Autodesk Inventor part; units mm, degrees
ref_plane "YZ Plane" through (0, 0, 0) normal (1, 0, 0) x (0, 1, 0)
ref_plane "XZ Plane" through (0, 0, 0) normal (0, 1, 0) x (-1, 0, 0)
ref_plane "XY Plane" through (0, 0, 0) normal (0, 0, 1) x (1, 0, 0)
sketch "Sketch1" plane through (0, 0, 0) normal (0, 1, 0) x (-1, 0, 0)
  line L0 (0, 0) -> (0, -45)
  line L1 (0, -45) -> (35, -45)
  line L2 (35, -45) -> (35, -49)
  line L3 (35, -49) -> (-4, -49)
  line L4 (-4, -49) -> (-4, 0)
  line L5 (-4, 0) -> (0, 0)
  dimension "d0" = 45
  dimension "d1" = 35
  dimension "d2" = 4
  dimension "d3" = 39
extrude "Extrusion1" add sketch "Sketch1" along normal blind 21
sketch "Sketch2" plane through (4, 0, 0) normal (1, 0, 0) x (0, 0, -1)
  line L0 (0, 21) -> (49, 21)
  line L1 (0, 21) -> (12.5, 21)
  line L2 (12.5, 21) -> (12.5, 16)
  line L3 (12.5, 16) -> (0, 16)
  line L4 (0, 16) -> (0, 21)
  line L5 (12.5, 16) -> (23.5, 16)
  line L6 (23.5, 16) -> (23.5, 5)
  line L7 (23.5, 5) -> (12.5, 5)
  line L8 (12.5, 5) -> (12.5, 16)
  circle A0 centre (12.5, 16) radius 1.5
  circle A1 centre (23.5, 16) radius 1.5
  circle A2 centre (12.5, 5) radius 1.5
  circle A3 centre (23.5, 5) radius 1.5
  point P0 (0, 0)
  dimension "d6" = 12.5
  dimension "d7" = 5
  dimension "d8" = 11
  dimension "d9" = 11
  dimension "d10" = 3
  dimension "d11" = 3
  dimension "d12" = 3
  dimension "d13" = 3
extrude "Extrusion2" cut sketch "Sketch2" against normal blind 21 contours A0 L5 L2 | L2 L3 A0 | L3 L8 A0 | L5 A0 L8 | A1 L6 L5 | L5 L6 A1 | A2 L7 L8 | L8 L7 A2 | A3 L7 L6 | L6 L7 A3
sketch "Sketch3" plane through (-35, 0, -45) normal (0, 0, 1) x (1, 0, 0)
  line L0 (0, 0) -> (0, 21)
  line L1 (0, 10.5) -> (10.5, 10.5)
  circle A0 centre (10.5, 10.5) radius 10.5
  line L2 (0, 21) -> (10.5, 21)
  line L3 (10.5, 21) -> (10.5, 0)
  line L4 (10.5, 0) -> (0, 0)
  line L5 (0, 0) -> (0, 21)
  circle A1 centre (10.5, 10.5) radius 8
  circle A2 centre (10.5, 10.5) radius 6.5
  line L6 (10.5, 18.5) -> (10.5, 17)
  line L7 (10.5, 4) -> (10.5, 2.5)
  line L8 (2.5, 10.5) -> (4, 10.5)
  line L9 (10.5, 10.5) -> (18.5, 10.5)
  line L10 (18.5, 10.5) -> (17, 10.5)
  circle A3 centre (10.5, 17.75) radius 1.1
  circle A4 centre (3.25, 10.5) radius 1.1
  circle A5 centre (17.75, 10.5) radius 1.1
  circle A6 centre (10.5, 3.25) radius 1.1
  circle A7 centre (10.5, 10.5) radius 3
  point P0 (35, 0)
  point P1 (10.5, 21)
  dimension "d16" = 10.5
  dimension "d17" = 16
  dimension "d18" = 13
  dimension "d19" = 2.2
  dimension "d20" = 2.2
  dimension "d21" = 2.2
  dimension "d22" = 2.2
  dimension "d23" = 6
extrude "Extrusion3" cut sketch "Sketch3" against normal blind 21 contours L0 A0 L4 | L0 L2 A0 | A4 A1 L1 | L1 A1 A4 | A6 A1 L3 | L3 A1 A6 | A1 A4 A2 L1 | L1 A2 A4 A1 | A3 A1 L3 | L3 A1 A3 | A1 A6 A2 L3 | L3 A2 A6 A1 | A2 A4 L1 | L1 A4 A2 | A1 L3 A2 A3 | A1 A3 A2 L3 | A2 A6 L3 | L3 A6 A2 | A5 A2 L9 A1 | A1 A5 | A2 L3 A3 | A2 A3 L3 | A1 L9 A2 A5 | A5 L9 A2 | A7 L3 L1 | L1 L3 A7 | A2 L9 A5 | L3 L9 A7 | L3 A7 L9
fillet "Fillet1" radius 4 1 edges at (0, 10.5, -45)
properties part number "L2"
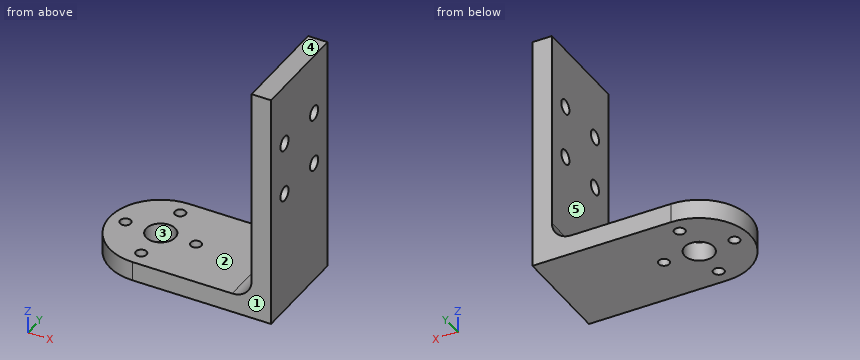
The listing builds one solid part. Answer for the finished solid, in the listing's coordinates (mm). Face numbers are marked on the shaded views. A direction names the side the tool comes from. Coordinates: 2 decimals unless noted, no trailing zeros. Loops run counter-clockwise (first coordinate to the right, second up) from the corner with the lowest first, then second, coordinate; pieces in that order, holes last. Notation, with made-up numbers: M -14,88 L 19,88 A19 ccw 19,106 Z; hole C -16.5,73.25 d8. An arc over 180 degrees is marked long. Answer as CSV lines item,"result". Start each with the question number.
(1) Find the intervals of material crossed by L1, parallel to X at y = 10.5, z = -47.15; L2, parallel to Y at x = -24.5, z = -46.5; L3, parallel to Y at x = 2.55, z = -23.5, in increasing order. Write a range as [from, to].
(2) The part is cut by section B-B (z = -12.5). Give the vertices of the cut face in (x, y).
(3) The part is cut by section C-C (x = -17.25). Give the vertices of the cut face in (y, z), and give its area (3 significant figures).
(4) Given pin 1 (2 mm diameter, centred on x = -31.75, y = 10.5, fed in from -Z); pin 2 (3 mm diameter, centred on x = -24.5, y = 3.25, fed in from +Z); pin 3 (12 mm diameter, centred on x = -7.5, y = 2, fed in from +Z); pin 4 (3.5 mm diameter, centred on y = 16, z = -12.5, fed in from -X), each flat-ended and moving along its own axis, determine where each tip first touches the part or whether it passes through.
(5) The part is cut by section A-A (y = 10.5). Give the vertices of the cut face in (x, z), and give its area (3 significant figures).
(6) For the marked faces 1 and 2, determine the directions among +Z, -Z, +X, -X, +Y, -Y from which every point of the face is accessible in a straight line to the end or side of a thin tool.
(7) The mould has two halves that part along X. Classify the marked faces 3, 4 and 5: pulls with the +X half, pulls with the -X half, needs draft (parallel to the pull), parting line crosses it, or undercut.
(8) The part is cut by section D-D (y = 19.5). Give the vertices of the cut face in (x, z), and give its area (3 significant figures).
Determined:
1,L1,"[-35, -32.85], [-30.65, -27.5], [-21.5, -18.35], [-16.15, 4]"
1,L2,"[0, 2.15], [4.35, 7.5], [13.5, 16.65], [18.85, 21]"
1,L3,"[0, 3.5], [6.5, 14.5], [17.5, 21]"
2,outline,"M 0,0 L 4,0 L 4,3.5 L 0,3.5 Z; M 0,6.5 L 4,6.5 L 4,14.5 L 0,14.5 Z; M 0,17.5 L 4,17.5 L 4,21 L 0,21 Z"
3,outline,"M 0,-49 L 9.4,-49 L 9.4,-45 L 0,-45 Z; M 11.6,-49 L 21,-49 L 21,-45 L 11.6,-45 Z"
3,area,"75.2 mm2"
4,pin 1,"through"
4,pin 2,"z = -45"
4,pin 3,"z = -44.12"
4,pin 4,"x = 0"
5,outline,"M -35,-49 L -32.85,-49 L -32.85,-45 L -35,-45 Z; M -30.65,-49 L -27.5,-49 L -27.5,-45 L -30.65,-45 Z; M -21.5,-49 L -18.35,-49 L -18.35,-45 L -21.5,-45 Z; M -16.15,-49 L 4,-49 L 4,0 L 0,0 L 0,-41 A4 cw -4,-45 L -16.15,-45 Z"
5,area,"298 mm2"
6,face 1,"+Z, -Z, +X, -X, -Y"
6,face 2,"+Z, -X, +Y, -Y"
7,face 3,"undercut"
7,face 4,"needs draft"
7,face 5,"pulls with the -X half"
8,outline,"M -29.91,-49 L 4,-49 L 4,0 L 0,0 L 0,-41 A4 cw -4,-45 L -29.91,-45 Z"
8,area,"319 mm2"
